Design review of the part built by this model. Coordinates are the model's own, in mm. A direction names the side the tool comes from. Round coordinates to 2 decimals unless told otherwise and drop trailing zeros. Loops run counter-clockwise (first coordinate to the right, second up) from the corner with the lowest first, then second, coordinate; pieces in that order, holes last. Notation, with made-up numbers: (-22, 16.25) -> (2, 16.25) arc R15 ccw to (2, 43.25) -> close; hole circle Ø8 at (-19.75, 80.25). An arc over 180 degrees is marked (long way). Use a Markdown table: item, result. Add a question column.
from build123d import *

# Parameters (mm, degrees)
F0_W     = 76.2
F0_H     = 127
F1_DEPTH = 25.4
F2_W     = 76.2
F2_H     = 50.8
F3_DEPTH = 25.4
F5_D     = 19.05
F6_R     = 25.4
F7_SIZE  = 2.54
F8_T     = -2.54


with BuildPart() as f1:
    # F0 (on Front) → F1 (new body)
    with BuildSketch(Plane.XZ):
        Rectangle(F0_W, F0_H)
    extrude(amount=F1_DEPTH)

    # F2 (on face) → F3 (join)
    with BuildSketch(Plane.XZ.offset(25.4)):
        with Locations((0, -38.1)):
            Rectangle(F2_W, F2_H)
    extrude(amount=F3_DEPTH)

    # F5 (through all)
    with Locations(Plane.XZ.offset(25.4)):
        with Locations((-19.05, 44.45), (19.05, 44.45)):
            Hole(F5_D / 2)

    # F6
    f6_edges = [f1.edges().sort_by_distance(p)[0] for p in [
        (38.1, -12.7, 63.5),
        (38.1, -38.1, -12.7),
    ]]
    fillet(f6_edges, radius=F6_R)

    # F7
    f7_edges = [f1.edges().sort_by_distance(p)[0] for p in [
        (-12.7, -25.4, 63.5),
        (-12.7, -50.8, -12.7),
    ]]
    chamfer(f7_edges, length=F7_SIZE)

    # F8
    f8_openings = [f1.faces().sort_by_distance(p)[0] for p in [
        (-0.03107, -25.379522, -63.5),
        (-0.500566, 0, -3.71782),
    ]]
    offset(amount=F8_T, openings=f8_openings, kind=Kind.INTERSECTION)


solid = f1.part
1. Mouldability with a two-part tool opening along X and no side actions: class faces 1 (the face through (-38.1, -19, -15)), 2 (the face through (38.1, -13, -25)), 3 (the face through (-13.06, -49.51, -13.95)), 4 (the face through (-35.56, -18, -16)) as +X half, -X half, draft (parallel to the pull), parting line (faces both ways), or undercut.
2. Consider section B-B on x = -19.05. State the section outline as (y, z) points (3 decimals), plus the area to 3 significant figures.
3. Consider section A-A on y = -13. State the section outline as (x, z) points (3 decimals), plus the area to 3 significant figures.
4. To check wall thickness, follow probe 1 along Z at (x, y) = (-19.05, -9) (3 decimals); probe 2 along Z at (x, y) = (19.05, -16) (3 decimals); probe 3 along X at (y, z) = (-39.5, -52). State the ranges of each line that lie inside material, in increasing order. Write a range as from..to.
5. For faces 5 (the face through (28.686, -34.686, -21.759)), 6 (the face through (36.81, -24.15, 0.53)), 7 (the face through (-13, -37, -12.7)), list the 3-axis set-ups (+Z, -Z, +X, -X, +Y, -Y) from which the entire face can be reached by the end or side of a thin tool; tool diameter is ignored.
6. Insertion check: P1, Ø11.5, axis at x = -19.05, z = 44.45, coming from the +Y side; P2, Ø1, axis at x = 3, z = 5, coming from the -Y side; P3, Ø7.5, axis at x = -23, y = -36, coming from the -Z side; P4, Ø17.5, axis at x = -22.5, y = -10, coming from the -Z side (3 decimals). Each pin has a flat end and moves straight along its axis. Give the tip position at first contact, or say it passes through.
7. Consider section C-C on z = 17.5. State the section outline as (x, y) points, plus the area to 3 significant figures.
8. Consider section D-D on y = -37.5. State the section outline as (x, z) points.
Verdict:
| question | item | result |
|---|---|---|
| 1 | face 1 | -X half |
| 1 | face 2 | +X half |
| 1 | face 3 | draft |
| 1 | face 4 | undercut |
| 2 | outline | (-50.8, -63.5) -> (-48.26, -63.5) -> (-48.26, -16.292) -> (-47.208, -15.24) -> (-22.86, -15.24) -> (-22.86, 32.385) -> (0, 32.385) -> (0, 34.925) -> (-25.4, 34.925) -> (-25.4, -12.7) -> (-48.26, -12.7) -> (-50.8, -15.24) -> close; (-25.4, 53.975) -> (0, 53.975) -> (0, 56.515) -> (-22.86, 56.515) -> (-22.86, 59.908) -> (-21.808, 60.96) -> (0, 60.96) -> (0, 63.5) -> (-22.86, 63.5) -> (-25.4, 60.96) -> close |
| 2 | area | 508 mm² |
| 3 | outline | (-38.1, -63.5) -> (-35.56, -63.5) -> (-35.56, 60.96) -> (12.7, 60.96) arc R22.86 cw to (35.56, 38.1) -> (35.56, -63.5) -> (38.1, -63.5) -> (38.1, 38.1) arc R25.4 ccw to (12.7, 63.5) -> (-38.1, 63.5) -> close; circle Ø24.13 at (-19.05, 44.45); circle Ø24.13 at (19.05, 44.45); hole circle Ø19.05 at (-19.05, 44.45); hole circle Ø19.05 at (19.05, 44.45) |
| 3 | area | 1,140 mm² |
| 4 | probe 1 | z = 32.385..34.925, 53.975..56.515, 60.96..63.5 |
| 4 | probe 2 | z = 32.385..34.925, 53.975..56.515, 60.06..62.693 |
| 4 | probe 3 | x = -38.1..-35.56, 35.56..38.1 |
| 5 | face 5 | -Z, +Y |
| 5 | face 6 | +Z, +X, -Y |
| 5 | face 7 | +Z, +X, -X, -Y |
| 6 | P1 | passes through |
| 6 | P2 | stops at y = -25.4 |
| 6 | P3 | stops at z = -15.24 |
| 6 | P4 | stops at z = 32.385 |
| 7 | outline | (-38.1, -25.4) -> (35.56, -25.4) -> (38.1, -22.86) -> (38.1, 0) -> (35.56, 0) -> (35.56, -21.81) -> (34.51, -22.86) -> (-35.56, -22.86) -> (-35.56, 0) -> (-38.1, 0) -> close |
| 7 | area | 307 mm² |
| 8 | outline | (-38.1, -63.5) -> (-35.56, -63.5) -> (-35.56, -15.24) -> (12.7, -15.24) arc R22.86 cw to (35.56, -38.1) -> (35.56, -63.5) -> (38.1, -63.5) -> (38.1, -38.1) arc R25.4 ccw to (12.7, -12.7) -> (-38.1, -12.7) -> close |
